Can you work these out from the model? Positions are in its coordinate system, mm. Round coordinates to 2 decimals unless told otherwise and drop trailing zeros. Order: outer loops, then holes, each group sorted by start corner. A loop starts at its lowest first (then second) coordinate and runs counter-clockwise, first axis right, second up. Notation, with made-up numbers: M 38.25,-0.75 L 54.25,-0.75 A34 cw 54.25,30.25 Z; hole C -35.5,55 d8. An arc over 180 degrees is marked long. Answer as a JSON object with one key per item and string values. Group by question number.
```python
from build123d import *

# Parameters (mm, degrees)
ESQUISSE1_W             = 60.96
ESQUISSE1_H             = 33.02
BOSS_EXTRU_1_DEPTH      = 14
ENL_V_MAT_EXTRU_1_REACH = 39.385
ESQUISSE2_R             = 2


with BuildPart() as part:
    # Esquisse1 → Boss.-Extru.1 (new body)
    with BuildSketch(Plane(origin=(0, 0, 0), x_dir=(1, 0, 0), z_dir=(0, 1, 0))):
        Rectangle(ESQUISSE1_W, ESQUISSE1_H)
    extrude(amount=BOSS_EXTRU_1_DEPTH)

    # Esquisse2 → Enlèv. mat.-Extru.1 (cut, up to next)
    with BuildSketch(Plane(origin=(0, 14, 0), x_dir=(1, 0, 0), z_dir=(0, 1, 0)), mode=Mode.PRIVATE) as enl_v_mat_extru_1_sk1:
        with Locations(Location((-28, 13.5, 0), (0, 0, 270))):
            Circle(ESQUISSE2_R)
    enl_v_mat_extru_1_tool1 = extrude(enl_v_mat_extru_1_sk1.sketch, amount=-ENL_V_MAT_EXTRU_1_REACH, mode=Mode.PRIVATE) & part.part
    # Esquisse2 → Enlèv. mat.-Extru.1 (cut, up to next)
    with BuildSketch(Plane(origin=(0, 14, 0), x_dir=(1, 0, 0), z_dir=(0, 1, 0)), mode=Mode.PRIVATE) as enl_v_mat_extru_1_sk2:
        with Locations(Location((28, 13.5, 0), (0, 0, 270))):
            Circle(ESQUISSE2_R)
    enl_v_mat_extru_1_tool2 = extrude(enl_v_mat_extru_1_sk2.sketch, amount=-ENL_V_MAT_EXTRU_1_REACH, mode=Mode.PRIVATE) & part.part
    # Esquisse2 → Enlèv. mat.-Extru.1 (cut, up to next)
    with BuildSketch(Plane(origin=(0, 14, 0), x_dir=(1, 0, 0), z_dir=(0, 1, 0)), mode=Mode.PRIVATE) as enl_v_mat_extru_1_sk3:
        with Locations(Location((28, -13.5, 0), (0, 0, 270))):
            Circle(ESQUISSE2_R)
    enl_v_mat_extru_1_tool3 = extrude(enl_v_mat_extru_1_sk3.sketch, amount=-ENL_V_MAT_EXTRU_1_REACH, mode=Mode.PRIVATE) & part.part
    # Esquisse2 → Enlèv. mat.-Extru.1 (cut, up to next)
    with BuildSketch(Plane(origin=(0, 14, 0), x_dir=(1, 0, 0), z_dir=(0, 1, 0)), mode=Mode.PRIVATE) as enl_v_mat_extru_1_sk4:
        with Locations(Location((-28, -13.5, 0), (0, 0, 270))):
            Circle(ESQUISSE2_R)
    enl_v_mat_extru_1_tool4 = extrude(enl_v_mat_extru_1_sk4.sketch, amount=-ENL_V_MAT_EXTRU_1_REACH, mode=Mode.PRIVATE) & part.part
    add(enl_v_mat_extru_1_tool1.solids().sort_by_distance((-28, 14, -13.5))[0], mode=Mode.SUBTRACT)
    add(enl_v_mat_extru_1_tool2.solids().sort_by_distance((28, 14, -13.5))[0], mode=Mode.SUBTRACT)
    add(enl_v_mat_extru_1_tool3.solids().sort_by_distance((28, 14, 13.5))[0], mode=Mode.SUBTRACT)
    add(enl_v_mat_extru_1_tool4.solids().sort_by_distance((-28, 14, 13.5))[0], mode=Mode.SUBTRACT)


solid = part.part
```
1) If we section it at B-B on x = 28: Write out the boundary of the cut face in (y, z), plus the area to 3 significant figures.
2) If we section it at C-C on y = 10.25: Write out the boundary of the cut face in (x, z), plus the area to 3 significant figures.
3) We'd pull the mould along X, two halves only. Please class faces 1 (the face through (0, 7, 16.51)), 2 (the face through (-29.952, 7.098, -13.934)), 3 (the face through (-30.48, 7, 0)): +X half, -X half, draft (parallel to the pull), parting line (faces both ways), or undercut.
4) I need wall thicknesses on line 1 along X through (y, z) = (4, 13.5); line 2 along X through (y, z) = (4.75, -12); line 3 along Z through (x, y) = (-27, 2.75). Which ranges of each line are inside material? Lowest first, please.
5) If we section it at A-A on z = -13.5: Write out the boundary of the cut face in (x, y), plus the area to 3 significant figures.
6) For pin 1 (3 mm diameter, centred on x = -28, z = 13.5, fed in from -Y), with a flat end and sliding along its axis, tell me the tip position at first contact or that it passes through.
Findings:
{
 "1": {"outline": "M 0,-16.51 L 14,-16.51 L 14,-15.5 L 0,-15.5 Z; M 0,-11.5 L 14,-11.5 L 14,11.5 L 0,11.5 Z; M 0,15.5 L 14,15.5 L 14,16.51 L 0,16.51 Z", "area": "350 mm^2"},
 "2": {"outline": "M -30.48,-16.51 L 30.48,-16.51 L 30.48,16.51 L -30.48,16.51 Z; hole C -28,-13.5 d4; hole C -28,13.5 d4; hole C 28,-13.5 d4; hole C 28,13.5 d4", "area": "1,960 mm^2"},
 "3": {"face 1": "draft", "face 2": "undercut", "face 3": "-X half"},
 "4": {"line 1": "x = -30.48 to -30, -26 to 26, 30 to 30.48", "line 2": "x = -30.48 to -29.32, -26.68 to 26.68, 29.32 to 30.48", "line 3": "z = -16.51 to -15.23, -11.77 to 11.77, 15.23 to 16.51"},
 "5": {"outline": "M -30.48,0 L -30,0 L -30,14 L -30.48,14 Z; M -26,0 L 26,0 L 26,14 L -26,14 Z; M 30,0 L 30.48,0 L 30.48,14 L 30,14 Z", "area": "741 mm^2"},
 "6": {"pin 1": "passes through"}
}
